The listing builds one solid part. Answer for the finished solid, in the listing's coordinates (mm). Round coordinates to 2 decimals unless told otherwise and drop trailing zeros. Write each loop counter-clockwise with the first axis right and the second up, starting at its lowest first coordinate (ties: lowest second). Pieces come first, ordered by that corner, then holes. Notation, with made-up numbers: M 32.5,30.25 L 36.5,30.25 A20 ccw 36.5,66.25 Z; hole C 39.25,-1.75 d1. An arc over 180 degrees is marked long. Answer as CSV lines item,"result". Start each with the question number.
Autodesk Inventor part; units mm, degrees
ref_plane "YZ Plane" through (0, 0, 0) normal (1, 0, 0) x (0, 1, 0)
ref_plane "XZ Plane" through (0, 0, 0) normal (0, 1, 0) x (-1, 0, 0)
ref_plane "XY Plane" through (0, 0, 0) normal (0, 0, 1) x (1, 0, 0)
sketch "Sketch2" plane through (0, 0, 0) normal (1, 0, 0) x (0, 1, 0)
  line L0 (0, 0) -> (1330, 0)
  line L1 (1330, 0) -> (1330, -50)
  line L2 (1330, -50) -> (0, -50)
  line L3 (0, -50) -> (0, 0)
  line L4 (1330, -50) -> (1293.2713, 0) construction
  line L5 (1330, 0) -> (1243.3333, -50)
  line L6 (0, 0) -> (28.8462, -50)
  dimension "d28" = 1330
  dimension "d29" = 50
  dimension "d31" = 36.3
  dimension "d32" = 60.018
  dimension "d36" = 60.018
extrude "Plate2" add sketch "Sketch2" along normal blind 3 contours L0 L5 L2 L6
chamfer "Corner Chamfer1" distance 3 angle 45 2 edges at (1.5, 1330, 0) (1.5, 0, 0)
fillet "Corner Round1" radius 6 2 edges at (1.5, 28.8462, -50) (1.5, 1243.3333, -50)
sketch "Sketch3" plane through (3, 0, 0) normal (1, 0, 0) x (0, 0, -1)
  line L0 (24, 397.5) -> (50, 397.5)
  line L1 (50, 397.5) -> (50, 400.5)
  line L2 (50, 400.5) -> (24, 400.5)
  line L3 (24, 400.5) -> (24, 397.5)
  line L4 (50, 1241.7267) -> (50, 32.3115)
  line L5 (50, 399) -> (0, 399) construction
  line L6 (0, 3) -> (0, 1327)
  line L7 (50, 798) -> (0, 798) construction
  line L8 (24, 796.5) -> (50, 796.5)
  line L9 (50, 796.5) -> (50, 799.5)
  line L10 (50, 799.5) -> (24, 799.5)
  line L11 (24, 799.5) -> (24, 796.5)
  point P0 (0, 0)
  point P1 (50, 796.5)
  point P2 (50, 799.5)
  dimension "d39" = 26
  dimension "d40" = 3
  dimension "d41" = 399
  dimension "d42" = 798
  dimension "d43" = 3
  dimension "d44" = 26
extrude "Extrusion1" cut sketch "Sketch3" against normal through all
sketch "Sketch4" plane through (3, 0, 0) normal (1, 0, 0) x (0, 0, -1)
  line L0 (15.0943, 691.214) -> (35.8481, 691.214) construction
  line L1 (35.8481, 691.214) -> (35.8481, 467.4424) construction
  line L2 (35.8481, 467.4424) -> (15.0943, 467.4424) construction
  line L3 (15.0943, 467.4424) -> (15.0943, 691.214) construction
  point P0 (0, 0)
mark "Mark1"
equation "\"d28\" = Конус_длина_борт"
equation "\"d32\" = Конус_Угол_борт"
equation "\"d36\" = Конус_Угол_борт"
equation "\"d40\" = Thickness"
equation "\"d43\" = Thickness"
equation "\"d44\" = d39"
equation "\"d30\" = Thickness"
equation "\"GapSize\" = Thickness"
equation "\"MinimumRemnant\" = 2 * Thickness"
equation "\"BendReliefDepth\" = 0.5 * Thickness"
equation "\"BendReliefWidth\" = Thickness"
equation "\"CornerReliefSize\" = 4 * Thickness"
equation "\"JacobiRadiusSize\" = BendRadius"
equation "\"TransitionRadius\" = BendRadius"
equation "\"Конус_длина_борт\" = 1330"
properties part number "MSC 110 STRINGER CONE" material "Stainless Steel"
Q1. Each of these flat-tipped pins is pushed along its axis until it touches: P1, Ø0.9, axis at x = 1, z = -43.5, coming from the -Y side; P2, Ø0.9, axis at x = 1, z = -40, coming from the +Y side; P3, Ø1.5, axis at x = 1, z = -31, coming from the -Y side. Where does it stop, or does it pass through?
Q2. Find section B-B (x = 2). Determine the outline of the cut face in (y, z).
Q3. Find section A-A (z = -33). Determine the outline of the cut face in (x, y), plus the area to 3 significant figures.
Q4. Straight lines are drawn through the part: L1, parallel to Y at x = 0.35, z = -26; L2, parallel to Y at x = 1.25, z = -44; L3, parallel to Y at x = 0.6, z = -12.5. For each, find the intervals that lie inside material, in ascending order.
Reported:
1,P1,"stops at y = 24.84"
1,P2,"stops at y = 1261.45"
1,P3,"stops at y = 17.45"
2,outline,"M 1.5,-2.6 L 27.11,-47 A6 ccw 32.31,-50 L 397.5,-50 L 397.5,-24 L 400.5,-24 L 400.5,-50 L 796.5,-50 L 796.5,-24 L 799.5,-24 L 799.5,-50 L 1241.73,-50 A6 ccw 1244.72,-49.2 L 1327.4,-1.5 L 1327,0 L 3,0 Z"
3,outline,"M 0,19.04 L 3,19.04 L 3,397.5 L 0,397.5 Z; M 0,400.5 L 3,400.5 L 3,796.5 L 0,796.5 Z; M 0,799.5 L 3,799.5 L 3,1272.8 L 0,1272.8 Z"
3,area,"3,740 mm2"
4,L1,"y = 15 to 397.5, 400.5 to 796.5, 799.5 to 1284.93"
4,L2,"y = 25.38 to 397.5, 400.5 to 796.5, 799.5 to 1253.73"
4,L3,"y = 7.21 to 1308.33"
